Verification items for the finished model (mm, model axes). A direction names the side the tool comes from. Round coordinates to 2 decimals unless told otherwise and drop trailing zeros. Write each loop counter-clockwise with the first axis right and the second up, starting at its lowest first coordinate (ties: lowest second). Pieces come first, ordered by that corner, then holes. Notation, with made-up numbers: (72.5, -11) -> (98.5, -11) arc R11 ccw to (98.5, -2) -> close; hole circle Ø7 at (19.5, 53.5). An arc over 180 degrees is marked (long way). Answer as a JSON object with one key per item and string values. Group by question number.
(1) Gauge pin test, flat ends, axial feed: pin 1 Ø3 at (y, z) = (58.5, 20) entering from -X; pin 2 Ø3 at (x, y) = (7.5, 86.5) entering from +Z; pin 3 Ø1 at (y, z) = (21.5, 12) entering from -X; pin 4 Ø22 at (x, z) = (-29, -9) entering from -Y. Record the tip position at first contact, or that the pin passes through.
(2) Sectioned sample at A-A on z = -13.5. Record the cut outline in (x, y).
(3) Set-up check for faces 4 (the face through (62, 8.37, 19.52)), 5 (the face through (39, 11.501, 0)), 6 (the face through (67.3, 131, -1.7)), 7 (the face through (82.113, 55, 12)), 8 (the face through (28, 5.151, -28)): record each of +Z, -Z, +X, -X, +Y, -Y from which the full face is reachable in a straight line by a thin tool's end or side.
(4) Draft check along X on faces 1 (the face through (67.323, 73.255, 36.618)), 2 (the face through (-37.8, 11.501, -2.3)), 3 (the face through (-7.6, 26.7, 40.3)). Enter one of: released by +X, released by -X, zero draft, split by the parting line, or undercut.
(5) Scan lines: L1, parallel to Y at x = 3, z = -48.5; L2, parallel to Y at x = 53, z = -15; L3, parallel to Y at x = 71, z = -15.5. Record each from-to range of solid material in increasing order. Write a range as from..to.
```python
from build123d import *

# Parameters (mm, degrees)
SWEEP5_PROFILE_R    = 41.275
SHELL13_T           = -2.54
SKETCH19_R          = 65
BOSS_EXTRUDE1_DEPTH = 6.35
SKETCH20_R          = 38.1
CUT_EXTRUDE1_DEPTH  = 6.35
SKETCH28_R          = 1.5
CUT_EXTRUDE5_DEPTH  = 10
CIRPATTERN1_COUNT   = 8


with BuildPart() as part:
    # Sweep5: sweep along a path in Sketch4
    with BuildLine(Plane.XY) as sweep5_path:
        Line((1.313416864, 11.5007856), (1.313416864, 41.5007856))
        ThreePointArc((1.313416864, 41.5007856), (16.19239238, 77.421810084), (52.113416864, 92.3007856))
        Line((52.113416864, 92.3007856), (82.113416864, 92.3007856))
    # Sweep5 profile (on start of the path) → Sweep5 (sweep)
    with BuildSketch(Plane(origin=(1.313416864, 11.5007856, 0), x_dir=(1, 0, 0), z_dir=(0, 1, 0))):
        Circle(SWEEP5_PROFILE_R)
    sweep(path=sweep5_path.line)

    # Shell13
    shell13_openings = [part.faces().sort_by_distance(p)[0] for p in [
        (82.113416864, 92.3007856, 0),
        (1.313416864, 11.5007856, 0),
    ]]
    offset(amount=SHELL13_T, openings=shell13_openings, kind=Kind.INTERSECTION)

    # Sketch19 → Boss-Extrude1 (add)
    with BuildSketch(Plane.XZ.offset(-11.5007856)):
        Circle(SKETCH19_R)
    extrude(amount=BOSS_EXTRUDE1_DEPTH)

    # Sketch20 → Cut-Extrude1 (cut)
    with BuildSketch(Plane(origin=(0, 5.1507856, 0), x_dir=(-1, 0, 0), z_dir=(0, -1, 0))):
        with Locations(Location((0, 0, 0), (0, 0, 180))):
            Circle(SKETCH20_R)
    extrude(amount=-CUT_EXTRUDE1_DEPTH, mode=Mode.SUBTRACT)

    # Sketch28 → Cut-Extrude5 (cut)
    with BuildSketch(Plane.XZ.offset(-5.1507856)):
        with Locations((0, 56.25)):
            Circle(SKETCH28_R)
    cut_extrude5 = extrude(amount=-CUT_EXTRUDE5_DEPTH, mode=Mode.SUBTRACT)

    # CirPattern1: Cut-Extrude5 ×8 about axis
    cirpattern1_axis = Axis((0, 0, 0), (0, 1, 0))
    for i in range(1, CIRPATTERN1_COUNT):
        add(cut_extrude5.rotate(cirpattern1_axis, i * 360 / CIRPATTERN1_COUNT), mode=Mode.SUBTRACT)


solid = part.part
```
Computed values:
{
 "1": {"pin 1": "x = -33.97", "pin 2": "z = 39.76", "pin 3": "x = -38.33", "pin 4": "y = 5.15"},
 "2": {"outline": "(-63.58, 5.15) -> (-35.63, 5.15) -> (-35.63, 11.5) -> (-34.99, 11.5) -> (-34.99, 41.5) arc R87.11 cw to (52.11, 128.61) -> (82.11, 128.61) -> (82.11, 131.31) -> (52.11, 131.31) arc R89.8 ccw to (-37.69, 41.5) -> (-37.69, 11.5) -> (-63.58, 11.5) -> close; (35.63, 5.15) -> (63.58, 5.15) -> (63.58, 11.5) -> (40.32, 11.5) -> (40.32, 41.5) arc R11.8 cw to (52.11, 53.3) -> (82.11, 53.3) -> (82.11, 55.99) -> (52.11, 55.99) arc R14.49 ccw to (37.62, 41.5) -> (37.62, 11.5) -> (35.63, 11.5) -> close"},
 "3": {"face 4": "-Y", "face 5": "none", "face 6": "+X", "face 7": "+Z, -Z, +X, +Y, -Y", "face 8": "+Z, -Z, +X, -X, -Y"},
 "4": {"face 1": "zero draft", "face 2": "undercut", "face 3": "split by the parting line"},
 "5": {"L1": "5.15..11.5", "L2": "5.15..11.5, 53.85..56.59, 128.01..130.75", "L3": "54.05..56.8, 127.8..130.55"}
}
